Build history of the part. All positions in model axes, mm. A direction names the side the tool comes from. Coordinates: 2 decimals unless noted, no trailing zeros. Order: outer loops, then holes, each group sorted by start corner. A loop starts at its lowest first (then second) coordinate and runs counter-clockwise, first axis right, second up. Notation, with made-up numbers: M 89.5,79 L 133.5,79 A14 cw 133.5,106 Z; hole C 13,50 d8. An arc over 180 degrees is marked long. Write item = value, one per line. Start each with the question number.
Q1. Drill centre lines: probe 1 along Z at (x, y) = (-30, -53); probe 2 along X at (y, z) = (-8.5, 3); probe 3 along Y at (x, z) = (-7, 7). Where is each one in solid material? Low to high.
Q2. Band-saw the part on B-B on y = 0. Write the cut outline in (x, z).
Q3. Pin check, flat tips, straight feed: P1, Ø5, axis at x = -8.5, z = 23.5, coming from the -Y side; P2, Ø5, axis at x = 2, z = 24, coming from the +Y side (3 decimals); P3, Ø3, axis at x = -9, z = 26, coming from the +Y side. Stop position of each tip, or through.
Q4. Pull direction Y, two halves, no side cores. Call faces 4 (the face through (-10, -38.1, 22)), 5 (the face through (-12.7, -44, 22)), 6 (the face through (-13.77, -61.99, 0.18)): released by +Y, released by -Y, zero draft, split by the parting line, or undercut.
Q5. Band-saw the part on C-C on z = 25.4. Write the cut outline in (x, y) (3 decimals).
Q6. Band-saw the part on D-D on z = 2. Write the cut outline in (x, y), plus the area to 3 significant figures.
Q7. Band-saw the part on A-A on x = 0. Write the cut outline in (y, z) (3 decimals).
Q8. 3-axis set-ups, long thin cutter, end or side, ignore diameter. For faces 1 (the face through (12.7, -44, 22)), 2 (the face through (-12.7, 0, 0)), 3 (the face through (-0.089, -47.127, 23.693)): which of +Z, -Z, +X, -X, +Y, -Y reach the whole face in a straight line?
```python
from build123d import *

# Parameters (mm, degrees)
SKETCH1_R           = 63.5
BOSS_EXTRUDE1_DEPTH = 12.7
SKETCH3_W           = 6.35
SKETCH3_H           = 12.7
BOSS_EXTRUDE2_DEPTH = 19.05
SKETCH4_R           = 3.175
BOSS_EXTRUDE3_DEPTH = 12.7
SKETCH5_W           = 25.4
SKETCH5_H           = 25.4
CUT_EXTRUDE1_DEPTH  = 26.4


with BuildPart() as part:
    # Sketch1 → Boss-Extrude1 (new body, symmetric)
    with BuildSketch(Plane.XY):
        Circle(SKETCH1_R)
    extrude(amount=BOSS_EXTRUDE1_DEPTH, both=True)

    # Sketch3 → Boss-Extrude2 (add)
    with BuildSketch(Plane.XY.offset(12.7)):
        with Locations((-9.525, 44.45)):
            Rectangle(SKETCH3_W, SKETCH3_H)
        with Locations((9.525, 44.45)):
            Rectangle(SKETCH3_W, SKETCH3_H)
    boss_extrude2 = extrude(amount=BOSS_EXTRUDE2_DEPTH)

    # Sketch4 → Boss-Extrude3 (add)
    with BuildSketch(Plane(origin=(-6.35, 0, 0), x_dir=(0, 0, -1), z_dir=(1, 0, 0))):
        with Locations((-25.4, 44.45)):
            Circle(SKETCH4_R)
    boss_extrude3 = extrude(amount=BOSS_EXTRUDE3_DEPTH)

    # Mirror1: Boss-Extrude2, Boss-Extrude3 across plane
    add(boss_extrude2.mirror(Plane.ZX))
    add(boss_extrude3.mirror(Plane.ZX))

    # Sketch5 → Cut-Extrude1 (cut, through all)
    with BuildSketch(Plane.XY.offset(12.7)):
        Rectangle(SKETCH5_W, SKETCH5_H)
    extrude(amount=-CUT_EXTRUDE1_DEPTH, mode=Mode.SUBTRACT)


solid = part.part
```
Recorded:
q1.probe_1 = -12.7 to 12.7
q1.probe_2 = -62.93 to -12.7, 12.7 to 62.93
q1.probe_3 = -63.11 to -12.7, 12.7 to 63.11
q2.outline = M -63.5,-12.7 L -12.7,-12.7 L -12.7,12.7 L -63.5,12.7 Z; M 12.7,-12.7 L 63.5,-12.7 L 63.5,12.7 L 12.7,12.7 Z
q3.P1 = -50.8
q3.P2 = 47.625
q3.P3 = 50.8
q4.face_4 = undercut
q4.face_5 = zero draft
q4.face_6 = split by the parting line
q5.outline = M -12.7,-50.8 L -6.35,-50.8 L -6.35,-47.625 L 6.35,-47.625 L 6.35,-50.8 L 12.7,-50.8 L 12.7,-38.1 L 6.35,-38.1 L 6.35,-41.275 L -6.35,-41.275 L -6.35,-38.1 L -12.7,-38.1 Z; M -12.7,38.1 L -6.35,38.1 L -6.35,41.275 L 6.35,41.275 L 6.35,38.1 L 12.7,38.1 L 12.7,50.8 L 6.35,50.8 L 6.35,47.625 L -6.35,47.625 L -6.35,50.8 L -12.7,50.8 Z
q6.outline = C 0,0 d127; hole M -12.7,-12.7 L 12.7,-12.7 L 12.7,12.7 L -12.7,12.7 Z
q6.area = 12,000 mm2
q7.outline = M -63.5,-12.7 L -12.7,-12.7 L -12.7,12.7 L -63.5,12.7 Z; C -44.45,25.4 d6.35; M 12.7,-12.7 L 63.5,-12.7 L 63.5,12.7 L 12.7,12.7 Z; C 44.45,25.4 d6.35
q8.face_1 = +Z, +X, +Y, -Y
q8.face_2 = +Z, -Z
q8.face_3 = none
